from build123d import *

# Parameters (mm, degrees)
SKETCH1_R                           = 25
SKETCH1_R_2                         = 15.5
BOSS_EXTRUDE1_DEPTH                 = 30
SKETCH3_R                           = 25
BOSS_EXTRUDE2_DEPTH                 = 8
BOSS_EXTRUDE3_DEPTH                 = 50
CUT_EXTRUDE1_DEPTH                  = 103.849404471
CUT_EXTRUDE1_DEPTH_BACK             = 103.849404471
SKETCH6_R                           = 9.5
FILLET2_R                           = 10
CUT_EXTRUDE2_REACH                  = 104.849
CUT_EXTRUDE2_END_RADIUS             = 25
SKETCH7_R                           = 8.25
CUT_EXTRUDE2_DIRECTION_2_REACH      = 104.849
CUT_EXTRUDE2_DIRECTION_2_END_RADIUS = 15.5
SKETCH8_R                           = 6.25
CUT_EXTRUDE3_DEPTH                  = 103.849404626
CUT_EXTRUDE3_OTHER_WAY_DEPTH        = 1
CUT_EXTRUDE3_OTHER_WAY_TAPER        = 1
CUT_EXTRUDE4_REACH                  = 104.396
CUT_EXTRUDE4_END_RADIUS             = 15.5
SKETCH9_R                           = 3.25


with BuildPart() as part:
    # Sketch1 → Boss-Extrude1 (new body)
    with BuildSketch(Plane(origin=(0, 0, 0), x_dir=(1, 0, 0), z_dir=(0, 1, 0))):
        with Locations(Location((0, 0, 0), (0, 0, 270))):
            Circle(SKETCH1_R)
        with Locations(Location((0, 0, 0), (0, 0, 270))):
            Circle(SKETCH1_R_2, mode=Mode.SUBTRACT)
    extrude(amount=BOSS_EXTRUDE1_DEPTH)

    # Sketch3 → Boss-Extrude2 (add)
    with BuildSketch(Plane(origin=(0, 30, 0), x_dir=(1, 0, 0), z_dir=(0, 1, 0))):
        with Locations(Location((0, 0, 0), (0, 0, 270))):
            Circle(SKETCH3_R)
    extrude(amount=BOSS_EXTRUDE2_DEPTH)

    # Sketch4 → Boss-Extrude3 (add)
    with BuildSketch(Plane(origin=(0, 38, 0), x_dir=(1, 0, 0), z_dir=(0, 1, 0))):
        with BuildLine():
            Line((-12, -21.931712199), (-12, 21.931712199))
            ThreePointArc((-12, 21.931712199), (-17.728160463, 17.627033971), (-22, 11.874342087))
            Line((-22, 11.874342087), (-22, -11.874342087))
            ThreePointArc((-22, -11.874342087), (-17.728160463, -17.627033971), (-12, -21.931712199))
        make_face()
        with BuildLine():
            ThreePointArc((22, 11.874342087), (17.728160463, 17.627033971), (12, 21.931712199))
            Line((12, 21.931712199), (12, -21.931712199))
            ThreePointArc((12, -21.931712199), (17.728160463, -17.627033971), (22, -11.874342087))
            Line((22, -11.874342087), (22, 11.874342087))
        make_face()
    extrude(amount=BOSS_EXTRUDE3_DEPTH)

    # Sketch6 → Cut-Extrude1 (cut, two sides: drawn at the far end of the back side and taken through both)
    with BuildSketch(Plane.ZY.offset(22).offset(-CUT_EXTRUDE1_DEPTH_BACK)):
        with Locations(Location((0, 70, 0), (0, 0, 180))):
            Circle(SKETCH6_R)
    extrude(amount=CUT_EXTRUDE1_DEPTH + CUT_EXTRUDE1_DEPTH_BACK, mode=Mode.SUBTRACT)

    # Fillet2
    # the kernel refuses this fillet: 10 mm, written as the material it adds along each edge
    with BuildSketch(Plane(origin=(-22, 38, -36.874342087), x_dir=(-1, 0, 0), z_dir=(0, 0, 1))) as fillet2_piece_1_section:
        with BuildLine():
            CenterArc((FILLET2_R, -FILLET2_R), FILLET2_R, 90, 90)
            Line((0, -FILLET2_R), (0, 0))
            Line((0, 0), (FILLET2_R, 0))
        make_face()
    fillet2_piece_1 = extrude(amount=73.748684174, mode=Mode.PRIVATE)
    fillet2_piece_1 = fillet2_piece_1 & Plane(origin=(0, 41.226834709, 0), x_dir=(0, 0, 1), z_dir=(0, -1, 0)) * Cylinder(25, 188, mode=Mode.PRIVATE)
    add(fillet2_piece_1)
    with BuildSketch(Plane(origin=(-12, 38, 46.931712199), x_dir=(1, 0, 0), z_dir=(0, 0, -1))) as fillet2_piece_2_section:
        with BuildLine():
            CenterArc((FILLET2_R, -FILLET2_R), FILLET2_R, 90, 90)
            Line((0, -FILLET2_R), (0, 0))
            Line((0, 0), (FILLET2_R, 0))
        make_face()
    fillet2_piece_2 = extrude(amount=93.863424399, mode=Mode.PRIVATE)
    fillet2_piece_2 = fillet2_piece_2 & Plane(origin=(0, 40.21683264, 0), x_dir=(0, 0, 1), z_dir=(0, -1, 0)) * Cylinder(25, 228, mode=Mode.PRIVATE)
    add(fillet2_piece_2)
    with BuildSketch(Plane(origin=(12, 38, -46.931712199), x_dir=(-1, 0, 0), z_dir=(0, 0, 1))) as fillet2_piece_3_section:
        with BuildLine():
            CenterArc((FILLET2_R, -FILLET2_R), FILLET2_R, 90, 90)
            Line((0, -FILLET2_R), (0, 0))
            Line((0, 0), (FILLET2_R, 0))
        make_face()
    fillet2_piece_3 = extrude(amount=93.863424399, mode=Mode.PRIVATE)
    fillet2_piece_3 = fillet2_piece_3 & Plane(origin=(0, 40.21683264, 0), x_dir=(0, 0, 1), z_dir=(0, -1, 0)) * Cylinder(25, 228, mode=Mode.PRIVATE)
    add(fillet2_piece_3)
    with BuildSketch(Plane(origin=(22, 38, 36.874342087), x_dir=(0, 1, 0), z_dir=(0, 0, -1))) as fillet2_piece_4_section:
        with BuildLine():
            CenterArc((FILLET2_R, FILLET2_R), FILLET2_R, 180, 90)
            Line((0, FILLET2_R), (0, 0))
            Line((0, 0), (FILLET2_R, 0))
        make_face()
    fillet2_piece_4 = extrude(amount=73.748684174, mode=Mode.PRIVATE)
    fillet2_piece_4 = fillet2_piece_4 & Plane(origin=(0, 41.226834878, 0), x_dir=(0, 0, 1), z_dir=(0, -1, 0)) * Cylinder(25, 188, mode=Mode.PRIVATE)
    add(fillet2_piece_4)

    # Cut-Extrude2: up to this cylinder (the profile starts inside it)
    cut_extrude2_end = Plane(origin=(0, 15, 0), z_dir=(0, -1, 0)) * Cylinder(CUT_EXTRUDE2_END_RADIUS, 260.698, mode=Mode.PRIVATE)
    # Sketch7 → Cut-Extrude2 (cut, up to the surface)
    with BuildSketch(Plane.ZY.offset(22), mode=Mode.PRIVATE) as cut_extrude2_sk1:
        with Locations((0, 15)):
            Circle(SKETCH7_R)
    cut_extrude2_tool1 = extrude(cut_extrude2_sk1.sketch, amount=CUT_EXTRUDE2_REACH, mode=Mode.PRIVATE) & cut_extrude2_end
    add(cut_extrude2_tool1.solids().sort_by_distance((-22, 15, 0))[0], mode=Mode.SUBTRACT)

    # Cut-Extrude2 direction 2: up to this cylinder (the profile starts outside it)
    cut_extrude2_direction_2_end = Plane(origin=(0, 15, 0), z_dir=(0, -1, 0)) * Cylinder(CUT_EXTRUDE2_DIRECTION_2_END_RADIUS, 241.698, mode=Mode.PRIVATE)
    # Sketch7 → Cut-Extrude2 direction 2 (cut, up to the surface)
    with BuildSketch(Plane.ZY.offset(22), mode=Mode.PRIVATE) as cut_extrude2_direction_2_sk1:
        with Locations((0, 15)):
            Circle(SKETCH7_R)
    cut_extrude2_direction_2_tool1 = extrude(cut_extrude2_direction_2_sk1.sketch, amount=-CUT_EXTRUDE2_DIRECTION_2_REACH, mode=Mode.PRIVATE) - cut_extrude2_direction_2_end
    add(cut_extrude2_direction_2_tool1.solids().sort_by_distance((-22, 15, 0))[0], mode=Mode.SUBTRACT)

    # Sketch8 → Cut-Extrude3 (cut)
    with BuildSketch(Plane(origin=(22, 0, 0), x_dir=(0, 0, -1), z_dir=(1, 0, 0))):
        with Locations(Location((0, 15, 0), (0, 0, 270))):
            Circle(SKETCH8_R)
    extrude(amount=CUT_EXTRUDE3_DEPTH, mode=Mode.SUBTRACT)

    # Sketch8 → Cut-Extrude3 other way (cut)
    with BuildSketch(Plane(origin=(22, 0, 0), x_dir=(0, 0, -1), z_dir=(1, 0, 0))):
        with Locations(Location((0, 15, 0), (0, 0, 270))):
            Circle(SKETCH8_R)
    extrude(amount=-CUT_EXTRUDE3_OTHER_WAY_DEPTH, taper=CUT_EXTRUDE3_OTHER_WAY_TAPER, mode=Mode.SUBTRACT)

    # Cut-Extrude4: up to this cylinder (the profile starts outside it)
    cut_extrude4_end = Plane(origin=(0, 15, 0), z_dir=(0, -1, 0)) * Cylinder(CUT_EXTRUDE4_END_RADIUS, 240.792, mode=Mode.PRIVATE)
    # Sketch9 → Cut-Extrude4 (cut, up to the surface)
    with BuildSketch(Plane(origin=(21, 0, 0), x_dir=(0, 0, -1), z_dir=(1, 0, 0)), mode=Mode.PRIVATE) as cut_extrude4_sk1:
        with Locations((0, 15)):
            Circle(SKETCH9_R)
    cut_extrude4_tool1 = extrude(cut_extrude4_sk1.sketch, amount=-CUT_EXTRUDE4_REACH, mode=Mode.PRIVATE) - cut_extrude4_end
    add(cut_extrude4_tool1.solids().sort_by_distance((21, 15, 0))[0], mode=Mode.SUBTRACT)


solid = part.part
The model under review builds one solid part; all positions refer to its coordinate system, in mm. A direction names the side the tool comes from. Round coordinates to 2 decimals unless told otherwise and drop trailing zeros. Loops run counter-clockwise (first coordinate to the right, second up) from the corner with the lowest first, then second, coordinate; pieces in that order, holes last. Notation, with made-up numbers: M 4,-17 L 33,-17 A18 ccw 33,16 Z; hole C -14,14.5 d5. An arc over 180 degrees is marked long. Answer as a JSON object with one key per item and string values.
Item 1: We need section D-D, the plane z = 0. State how many separate pieces and enclosed holes the cut face has, and give its area (3 significant figures).
Check sheet entries:
{"separate pieces": "5", "enclosed holes": "0", "area": "1,420 mm2"}
Item 2: We need section B-B, the plane y = 54. State the section outline as (x, z) points, and give its area (3 significant figures).
Check sheet entries:
{"outline": "M -22,-11.87 A25 ccw -12,-21.93 L -12,21.93 A25 ccw -22,11.87 Z; M 12,-21.93 A25 ccw 22,-11.87 L 22,11.87 A25 ccw 12,21.93 Z", "area": "715 mm2"}
Item 3: For line 1 along Y through (x, z) = (-15, -7); line 2 along X through (y, z) = (80.5, -4.5); line 3 along Y through (x, z) = (2, 0.5), list the stretches that pass through material, from the lowest coordinate up.
Check sheet entries:
{"line 1": "0 to 10.63, 19.37 to 63.58, 76.42 to 88", "line 2": "-22 to -12, 12 to 22", "line 3": "30 to 38"}
Item 4: The part is to be moulded in two halves that separate along Z. For faces 1 (the face through (-22, 59, 0)), 2 (the face through (-16.93, 63.58, 7)), say which applies: +Z half, -Z half, draft (parallel to the pull), parting line (faces both ways), or undercut.
Check sheet entries:
{"face 1": "draft", "face 2": "undercut"}
Item 5: We need section C-C, the plane x = 0. State the section outline as (y, z) points.
Check sheet entries:
{"outline": "M 0,-25 L 38,-25 L 38,25 L 0,25 L 0,15.5 L 30,15.5 L 30,-15.5 L 0,-15.5 Z"}
Item 6: Clearance check with flat-ended pins moving along their axes: P1, Ø3, axis at x = 0, z = 3.5, coming from the +Y side; P2, Ø19, axis at y = 67.5, z = 4, coming from the +X side; P3, Ø12, axis at y = 72, z = 0.5, coming from the -X side; P4, Ø10, axis at x = -6, z = -18.5, coming from the +Y side. State where each tip first meets the part, or that it passes through.
Check sheet entries:
{"P1": "y = 38", "P2": "x = 22", "P3": "through", "P4": "y = 43.64"}
Item 7: We need section A-A, the plane y = 70. State the section outline as (x, z) points, and give its area (3 significant figures).
Check sheet entries:
{"outline": "M -22,-11.87 A25 ccw -12,-21.93 L -12,-9.5 L -22,-9.5 Z; M -22,9.5 L -12,9.5 L -12,21.93 A25 ccw -22,11.87 Z; M 12,-21.93 A25 ccw 22,-11.87 L 22,-9.5 L 12,-9.5 Z; M 12,9.5 L 22,9.5 L 22,11.87 A25 ccw 12,21.93 Z", "area": "335 mm2"}
Item 8: Tool access review of faces 3 (the face through (8.99, 40.85, -0.35)), 4 (the face through (21.382, 9.049, -1.874)), 5 (the face through (22, 59, 0)): name each direction out of +Z, -Z, +X, -X, +Y, -Y from which nothing blocks a thin tool from reaching the whole face with its end or side.
Check sheet entries:
{"face 3": "+Z, -Z, +Y", "face 4": "+X", "face 5": "+Z, -Z, +X, +Y"}
